Job drawing, mm, ordinate dimensions from the low corner. One solid piece. Coordinates: 2 decimals unless noted, no trailing zeros. Write each loop counter-clockwise with the first axis right and the second up, starting at its lowest first coordinate (ties: lowest second). Pieces come first, ordered by that corner, then holes. Notation, with made-up numbers: (47.25, 35.5) - (70.25, 35.5) arc R35 ccw to (70.25, 70.5) - close; hole circle Ø11 at (-21, 86.5). An arc over 180 degrees is marked (long way). Put each result on its own line as item: value. Start each with the question number.
1. Saw through at A-A, the plane y = 57.15. Write the cut outline in (x, z) (1 decimal).
2. Drop flat-ended pins along their axis: P1, Ø5, axis at x = 12.5, z = 20.5, coming from the +Y side (1 decimal); P2, Ø10, axis at x = 66, z = 15, coming from the -Y side (1 decimal); P3, Ø12, axis at x = 75, y = 41.5, coming from the -Z side (3 decimals); P4, Ø4, axis at x = 44.45, z = 12.7, coming from the +Y side. Give the stop position or say it passes through.
3. Saw through at C-C, the plane x = 31.5. Write the cut outline in (y, z) (1 decimal), plus the area to 3 significant figures.
4. Saw through at D-D, the plane x = 44.45. Give the number of separate pieces and of enclosed holes in the cut face, plus the area to 3 significant figures.
5. Pull direction X, two halves, no side cores. Call the marked faces 1 and 2: released by +X, released by -X, zero draft, split by the parting line, or undercut.
6. Drill centre lines: L1, parallel to Y at x = 44.45, z = 24.4 (1 decimal); L2, parallel to X at y = 57, z = 18.5; L3, parallel to Z at x = 44.45, y = 12. Where is each one in solid material? Low to high. Write a range as from..to.
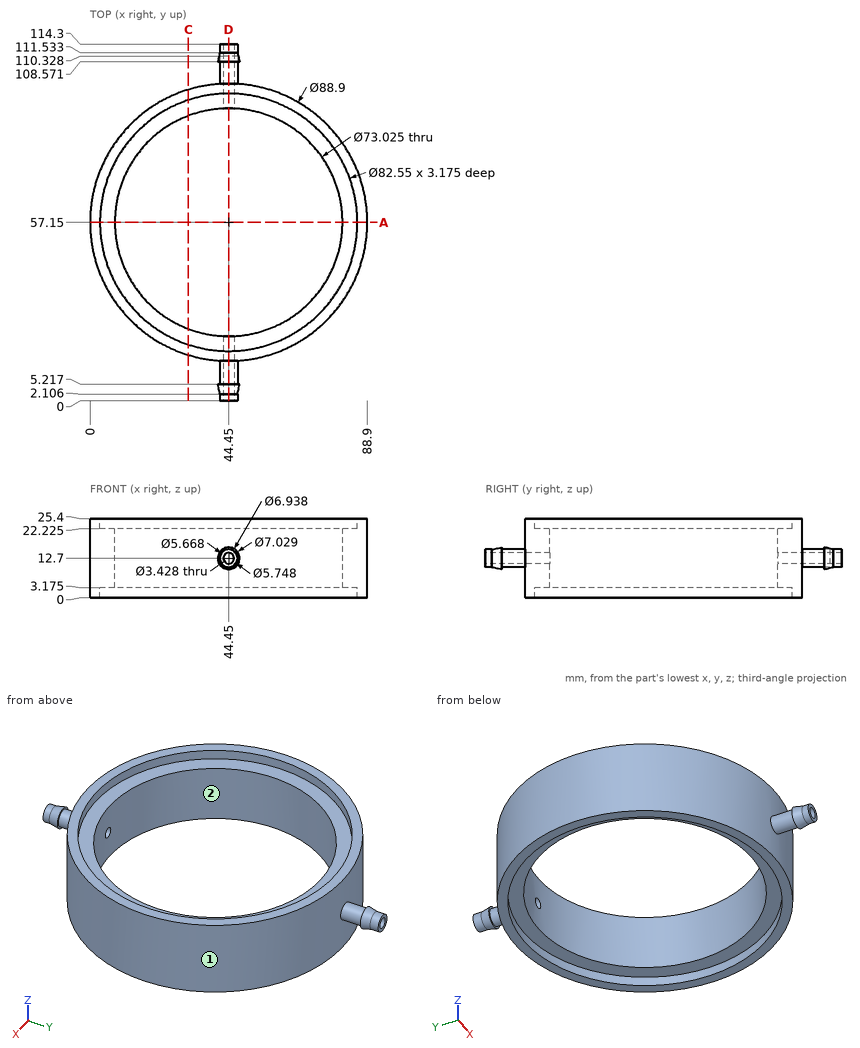
Final values:
1. outline: (0, 0) - (3.2, 0) - (3.2, 3.2) - (7.9, 3.2) - (7.9, 22.2) - (3.2, 22.2) - (3.2, 25.4) - (0, 25.4) - close; (81, 3.2) - (85.7, 3.2) - (85.7, 0) - (88.9, 0) - (88.9, 25.4) - (85.7, 25.4) - (85.7, 22.2) - (81, 22.2) - close
2. P1: stops at y = 90.4
2. P2: stops at y = 15.9
2. P3: stops at z = 3.175
2. P4: stops at y = 114.3
3. outline: (14.6, 0) - (18, 0) - (18, 3.2) - (23, 3.2) - (23, 22.2) - (18, 22.2) - (18, 25.4) - (14.6, 25.4) - close; (91.3, 3.2) - (96.3, 3.2) - (96.3, 0) - (99.7, 0) - (99.7, 25.4) - (96.3, 25.4) - (96.3, 22.2) - (91.3, 22.2) - close
3. area: 362 mm²
4. separate pieces: 4
4. enclosed holes: 0
4. area: 349 mm²
5. face 1: split by the parting line
5. face 2: undercut
6. L1: y = 12.7..15.9, 98.4..101.6
6. L2: x = 0..7.94, 80.96..88.9
6. L3: z = 9.87..10.99, 14.41..15.53
